For this review, use the dimensioned drawing (mm, ordinates from the lowest corner) and the shaded views. Coordinates: 2 decimals unless noted, no trailing zeros. Loops run counter-clockwise (first coordinate to the right, second up) from the corner with the lowest first, then second, coordinate; pieces in that order, holes last. Notation, with made-up numbers: M -8,-7 L 12,-7 A27 cw 12,28 Z; hole C 72,-35 d10. An arc over 180 degrees is marked long. Write each question's results on one line, items separated by ' | '. Start each with the question number.
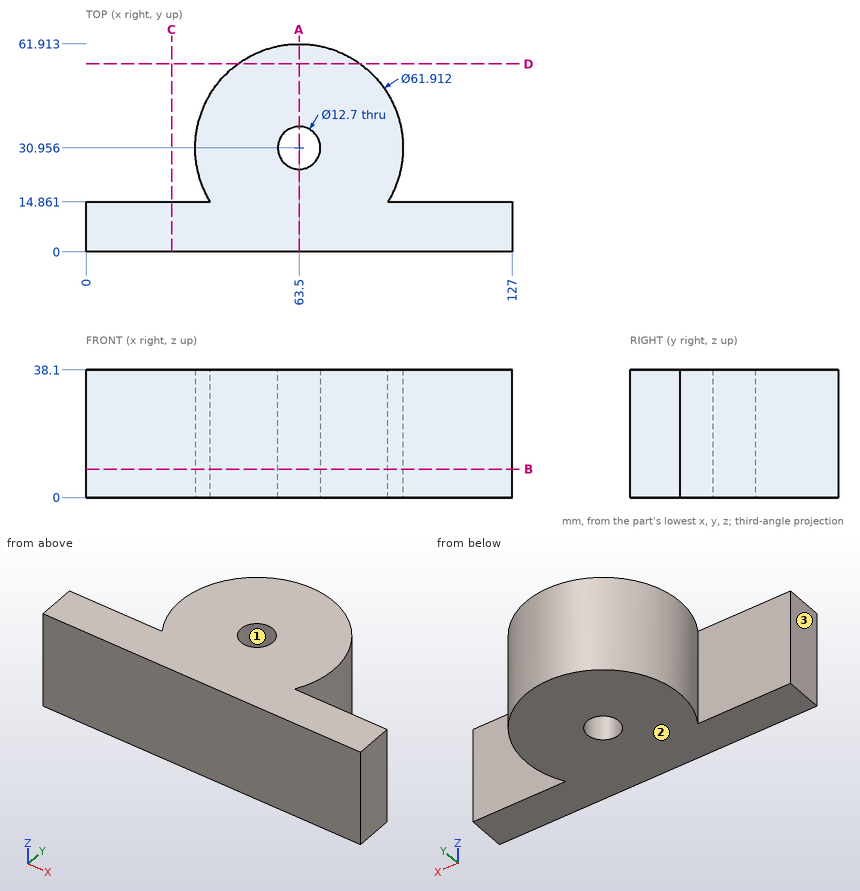
Q1. Insertion check: P1, Ø12, axis at x = 20.5, z = 23, coming from the +Y side; P2, Ø1.5, axis at y = 37, z = 26.5, coming from the +X side; P3, Ø7.5, axis at x = 63.5, y = 30.96, coming from the -Z side; P4, Ø2, axis at y = 55.5, z = 23.5, coming from the +X side. Each pin has a flat end and moves straight along its axis. Give the tip position at first contact, or say it passes through.
Q2. To check wall thickness, follow line 1 along Y through (x, z) = (63.5, 30); line 2 along X through (y, z) = (28, 3) (1 decimal); line 3 along Y through (x, z) = (110, 3). State the ranges of each line that lie inside material, in increasing order.
Q3. Take a section at D-D, the plane y = 56. Give the boundary of the cut face in (x, z), then the cut area to 3 significant figures.
Q4. Take a section at C-C, the plane x = 25.5. Give the boundary of the cut face in (y, z).
Q5. The part is to be moulded in two halves that separate along X. For the marked faces 1, 2 and 3, say which applies: pulls with the +X half, pulls with the -X half, needs draft (parallel to the pull), parting line crosses it, or undercut.
Q6. Take a section at B-B, the plane z = 8.5. Give the boundary of the cut face in (x, y).
Q7. Take a section at A-A, the plane x = 63.5. Give the boundary of the cut face in (y, z), then the cut area to 4 significant figures.
Results:
1) P1: y = 14.86 | P2: x = 94 | P3: through | P4: x = 83.6
2) line 1: 0 to 24.61, 37.31 to 61.91 | line 2: 32.7 to 57.9, 69.1 to 94.3 | line 3: 0 to 14.86
3) outline: M 45.3,0 L 81.7,0 L 81.7,38.1 L 45.3,38.1 Z | area: 1,390 mm^2
4) outline: M 0,0 L 14.86,0 L 14.86,38.1 L 0,38.1 Z
5) face 1: undercut | face 2: needs draft | face 3: pulls with the -X half
6) outline: M 0,0 L 127,0 L 127,14.86 L 89.94,14.86 A30.96 ccw long 37.06,14.86 L 0,14.86 Z; hole C 63.5,30.96 d12.7
7) outline: M 0,0 L 24.61,0 L 24.61,38.1 L 0,38.1 Z; M 37.31,0 L 61.91,0 L 61.91,38.1 L 37.31,38.1 Z | area: 1,875 mm^2
